The model under review builds one solid part; all positions refer to its coordinate system, in mm. A direction names the side the tool comes from. Coordinates: 2 decimals unless noted, no trailing zeros. Write each loop counter-clockwise with the first axis right and the second up, starting at its lowest first coordinate (ties: lowest second). Pieces come first, ordered by that corner, then holes. Notation, with made-up numbers: (77.25, 71) - (106.25, 71) arc R22 cw to (106.25, 80) - close; hole circle Ø10 at (60, 20.25). An arc over 180 degrees is marked (long way). Return JSON: item names as keys, results as strings. Group by question number.
(1) We need section B-B on z = -1. State the section outline as (x, y) points.
(2) To check wall thickness, follow L1, parallel to Y at x = 49, z = -8.5; L2, parallel to X at y = 12, z = -15; L3, parallel to Y at x = 28.5, z = -1. State the ranges of each line that lie inside material, in increasing order. Write a range as from..to.
(3) Draft analysis for pull direction X (two halves, no side actions). For faces 1 (the face through (0, 19, -11)), 2 (the face through (53.2, 28.07, -17.01)), 3 (the face through (27, 0, -2)), state which applies: released by +X, released by -X, zero draft, split by the parting line, or undercut.
(4) For pin 1 Ø3.5 at (x, y) = (51, 28) entering from -Z; pin 2 Ø1.5 at (y, z) = (27.5, -4.5) entering from -X; pin 3 Ø5 at (x, z) = (59, -9.5) entering from -Y; pin 4 Ø5 at (x, z) = (58.5, -7) entering from +Y, all flat-tipped, find the tip position at first contact; note any pin that passes through.
(5) We need section C-C on x = 32.5. State the section outline as (y, z) points.
(6) We need section A-A on y = 7. State the section outline as (x, z) points.
(7) We need section D-D on y = 3. State the section outline as (x, z) points.
(8) Tool access review of faces 4 (the face through (27, 1, -5.918)), 5 (the face through (59, 1, -10)), 6 (the face through (27, 34, -9)), 7 (the face through (59, 36.5, -8)), 8 (the face through (55.25, 9.5, -4.23)): name each direction out of +Z, -Z, +X, -X, +Y, -Y from which nothing blocks a thin tool from reaching the whole face with its end or side.
```python
from build123d import *

# Parameters (mm, degrees)
SKETCH_1_W                     = 18
SKETCH_1_H                     = 37
EXTRUDE_1_DEPTH                = 55.5
SKETCH_2_R                     = 5
CUT_EXTRUDE_1_DEPTH            = 0.5
CUT_EXTRUDE_START              = -0.5
SKETCH_3_R                     = 5
CUT_EXTRUDE_2_DEPTH            = 0.5
SKETCH_4_R                     = 1.5
CUT_EXTRUDE_3_DEPTH            = 70.088711089
SKETCH_5_W                     = 1.835428096
SKETCH_5_H                     = 2.75652024
CUT_EXTRUDE_4_DEPTH            = 70.088711089
SKETCH_6_W                     = 5
SKETCH_6_H                     = 17
CUT_EXTRUDE_5_DEPTH            = 70.088711089
SKETCH_7_W                     = 8
SKETCH_7_H                     = 12
CUT_EXTRUDE_6_DEPTH            = 70.088711089
SKETCH_8_R                     = 2.5
EXTRUDE_2_DEPTH                = 1.5
SKETCH_9_W                     = 17.5
SKETCH_9_H                     = 35.5
EXTRUDE_3_DEPTH                = 4.5
SKETCH_10_W                    = 7
SKETCH_10_H                    = 11
EXTRUDE_4_DEPTH                = 54
CUT_EXTRUDE_7_REACH            = 75.58
SKETCH_11_W                    = 4.5
SKETCH_11_H                    = 18.5
HOLE_WIZARD_M3_1_D             = 2.5
HOLE_WIZARD_M3_1_DEPTH         = 7.5
HOLE_WIZARD_M3_1_TIP           = 0.751075774
HOLE_WIZARD_M3_1_2_D           = 3.4
HOLE_WIZARD_M3_1_2_DEPTH       = 5
HOLE_WIZARD_M3_1_2_CBORE_D     = 6.5
HOLE_WIZARD_M3_1_2_CBORE_DEPTH = 3
CUT_EXTRUDE_8_REACH            = 75.704
SKETCH_16_R                    = 3


with BuildPart() as part:
    # 草图1 → 凸台-拉伸1 (new body)
    with BuildSketch(Plane(origin=(0, 0, 0), x_dir=(0, 0, -1), z_dir=(1, 0, 0))):
        with Locations((9, 18.5)):
            Rectangle(SKETCH_1_W, SKETCH_1_H)
    extrude(amount=EXTRUDE_1_DEPTH)

    # 草图2 → 切除-拉伸1 (cut)
    with BuildSketch(Plane.ZY):
        with Locations((-9, 11)):
            Circle(SKETCH_2_R)
    extrude(amount=-CUT_EXTRUDE_1_DEPTH, mode=Mode.SUBTRACT)

    # 草图3 → 切除-拉伸2 (cut)
    with BuildSketch(Plane(origin=(55.5, 0, 0), x_dir=(0, 0, -1), z_dir=(1, 0, 0)).offset(CUT_EXTRUDE_START)):
        with Locations(Location((9, 11, 0), (0, 0, 180))):
            Circle(SKETCH_3_R)
    extrude(amount=CUT_EXTRUDE_2_DEPTH, mode=Mode.SUBTRACT)

    # 草图4 → 切除-拉伸3 (cut, through all)
    with BuildSketch(Plane.ZY):
        with Locations((-13, 3)):
            Circle(SKETCH_4_R)
        with Locations(Location((-5, 3, 0), (0, 0, 180))):
            Circle(SKETCH_4_R)
    extrude(amount=-CUT_EXTRUDE_3_DEPTH, mode=Mode.SUBTRACT)

    # 草图5 → 切除-拉伸4 (cut, through all)
    with BuildSketch(Plane.ZY):
        with Locations((-13, 1.37826012)):
            Rectangle(SKETCH_5_W, SKETCH_5_H)
        with Locations((-5, 1.37826012)):
            Rectangle(SKETCH_5_W, SKETCH_5_H)
    extrude(amount=-CUT_EXTRUDE_4_DEPTH, mode=Mode.SUBTRACT)

    # 草图6 → 切除-拉伸5 (cut, through all)
    with BuildSketch(Plane.ZY):
        with Locations((-2.5, 28.5)):
            Rectangle(SKETCH_6_W, SKETCH_6_H)
    extrude(amount=-CUT_EXTRUDE_5_DEPTH, mode=Mode.SUBTRACT)

    # 草图7 → 切除-拉伸6 (cut, through all)
    with BuildSketch(Plane.ZY):
        with Locations((-9, 28)):
            Rectangle(SKETCH_7_W, SKETCH_7_H)
    extrude(amount=-CUT_EXTRUDE_6_DEPTH, mode=Mode.SUBTRACT)

    # 草图8 → 凸台-拉伸2 (add)
    with BuildSketch(Plane(origin=(55, 0, 0), x_dir=(0, 0, -1), z_dir=(1, 0, 0))):
        with Locations((9, 11)):
            Circle(SKETCH_8_R)
    extrude(amount=EXTRUDE_2_DEPTH)

    # 草图9 → 凸台-拉伸3 (add)
    with BuildSketch(Plane(origin=(56.5, 0, 0), x_dir=(0, 0, -1), z_dir=(1, 0, 0))):
        with Locations((8.25, 18.75)):
            Rectangle(SKETCH_9_W, SKETCH_9_H)
    extrude(amount=EXTRUDE_3_DEPTH)

    # 草图10 → 凸台-拉伸4 (add)
    with BuildSketch(Plane.ZY.offset(-56.5)):
        with Locations((-3, 28)):
            Rectangle(SKETCH_10_W, SKETCH_10_H)
    extrude(amount=EXTRUDE_4_DEPTH)

    # 草图11 → 切除-拉伸7 (cut, up to next)
    with BuildSketch(Plane(origin=(61, 0, 0), x_dir=(0, 0, -1), z_dir=(1, 0, 0)), mode=Mode.PRIVATE) as cut_extrude_7_sk1:
        with Locations((1.75, 10.25)):
            Rectangle(SKETCH_11_W, SKETCH_11_H)
    cut_extrude_7_tool1 = extrude(cut_extrude_7_sk1.sketch, amount=-CUT_EXTRUDE_7_REACH, mode=Mode.PRIVATE) & part.part
    add(cut_extrude_7_tool1.solids().sort_by_distance((61, 10.25, -1.75))[0], mode=Mode.SUBTRACT)

    # Hole Wizard M3 _1
    with Locations(Plane(origin=(61, 0, 0), x_dir=(0, 0, -1), z_dir=(1, 0, 0))):
        with Locations((13.5, 33), (3, 23)):
            Hole(HOLE_WIZARD_M3_1_D / 2, depth=HOLE_WIZARD_M3_1_DEPTH)
            with Locations((0, 0, -(HOLE_WIZARD_M3_1_DEPTH + HOLE_WIZARD_M3_1_TIP / 2))):  # 118° drill point
                Cone(0, HOLE_WIZARD_M3_1_D / 2, HOLE_WIZARD_M3_1_TIP, mode=Mode.SUBTRACT)

    # Hole Wizard M3 _1 2
    with Locations(Plane.XY.offset(-13)):
        with Locations((4, 28), (51.5, 28)):
            CounterBoreHole(HOLE_WIZARD_M3_1_2_D / 2, HOLE_WIZARD_M3_1_2_CBORE_D / 2, HOLE_WIZARD_M3_1_2_CBORE_DEPTH, depth=HOLE_WIZARD_M3_1_2_DEPTH)

    # 草图16 → 切除-拉伸8 (cut, up to next)
    with BuildSketch(Plane.XY.offset(0.5), mode=Mode.PRIVATE) as cut_extrude_8_sk1:
        with Locations((51, 28)):
            Circle(SKETCH_16_R)
    cut_extrude_8_tool1 = extrude(cut_extrude_8_sk1.sketch, amount=-CUT_EXTRUDE_8_REACH, mode=Mode.PRIVATE) & part.part
    add(cut_extrude_8_tool1.solids().sort_by_distance((51, 28, 0.5))[0], mode=Mode.SUBTRACT)


solid = part.part
```
Ans:
{
 "1": {"outline": "(0, 0) - (55.5, 0) - (55.5, 20) - (0, 20) - close; (2.5, 22.5) - (56.5, 22.5) - (56.5, 19.5) - (61, 19.5) - (61, 36.5) - (56.5, 36.5) - (56.5, 33.5) - (2.5, 33.5) - close; hole circle Ø6 at (51, 28)"},
 "2": {"L1": "0..22, 34..37", "L2": "0..55.5, 56.5..61", "L3": "0..20, 22.5..33.5"},
 "3": {"face 1": "released by -X", "face 2": "undercut", "face 3": "zero draft"},
 "4": {"pin 1": "z = -18", "pin 2": "x = 2.5", "pin 3": "y = 1", "pin 4": "y = 36.5"},
 "5": {"outline": "(0, -18) - (37, -18) - (37, -5) - (34, -5) - (34, -13) - (22, -13) - (22, -5) - (20, -5) - (20, 0) - (0, 0) - (0, -4.08) - (1.81, -4.08) arc R1.5 cw (long way) to (1.81, -5.92) - (0, -5.92) - (0, -12.08) - (1.81, -12.08) arc R1.5 cw (long way) to (1.81, -13.92) - (0, -13.92) - close; (22.5, -6.5) - (33.5, -6.5) - (33.5, 0.5) - (22.5, 0.5) - close"},
 "6": {"outline": "(0, -18) - (55.5, -18) - (55.5, -12) - (55, -12) - (55, -6) - (55.5, -6) - (55.5, 0) - (0, 0) - (0, -6) - (0.5, -6) - (0.5, -12) - (0, -12) - close; (56.5, -17) - (61, -17) - (61, -4) - (56.5, -4) - close"},
 "7": {"outline": "(0, -18) - (55.5, -18) - (55.5, -14.5) - (0, -14.5) - close; (0, -11.5) - (55.5, -11.5) - (55.5, -6.5) - (0, -6.5) - close; (0, -3.5) - (55.5, -3.5) - (55.5, 0) - (0, 0) - close; (56.5, -17) - (61, -17) - (61, -4) - (56.5, -4) - close"},
 "8": {"face 4": "-X, -Y", "face 5": "+Z, -Z, +X, -Y", "face 6": "+Z, -X", "face 7": "+Z, -Z, +X, +Y", "face 8": "none"}
}
